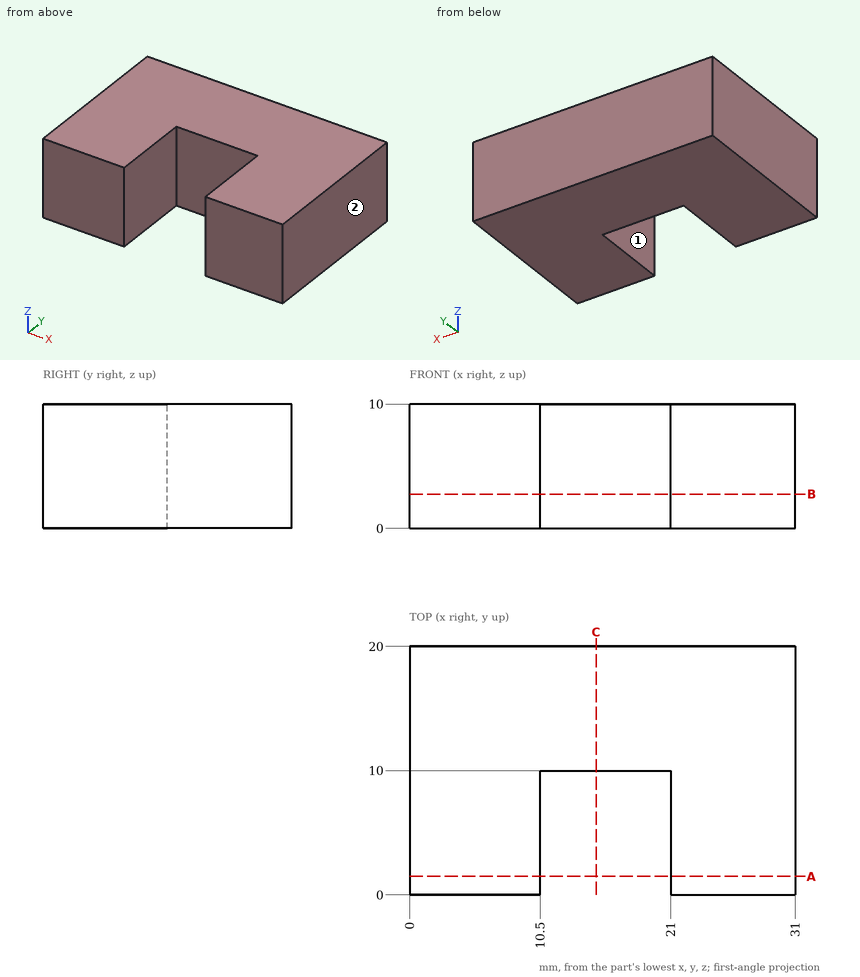
Verification items for this drawing (mm, ordinates from the low corner). A direction names the side the tool comes from. Give positions to 0.01 mm unless a question says otherwise; leave off trailing zeros. Order: outer loops, then holes, each group sorted by start corner. A loop starts at its lowest first (then second) coordinate and runs counter-clockwise, first axis right, second up.
1) Cross-section at A-A (y = 1.5). Record the boundary of the cut face in (x, z).
Results are:
outline: (0, 0) - (10.5, 0) - (10.5, 10) - (0, 10) - close; (21, 0) - (31, 0) - (31, 10) - (21, 10) - close
2) Cross-section at C-C (x = 15). Record the boundary of the cut face in (y, z), then the cut area to 3 significant figures.
Results are:
outline: (10, 0) - (20, 0) - (20, 10) - (10, 10) - close
area: 100 mm2
3) Material ranges on probe 1 along X at (y, z) = (6.5, 5); probe 2 along Y at (x, z) = (19.5, 4.5), recorded low to high.
Results are:
probe 1: x = 0 to 10.5, 21 to 31
probe 2: y = 10 to 20
4) Gauge pin test, flat end, axial feed: pin 1 (3 mm diameter, centred on x = 11.5, z = 3, fed in from -Y). Record the tip position at first contact, or that the pin passes through.
Results are:
pin 1: stops at y = 0
5) Cross-section at B-B (z = 2.75). Record the boundary of the cut face in (x, y).
Results are:
outline: (0, 0) - (10.5, 0) - (10.5, 10) - (21, 10) - (21, 0) - (31, 0) - (31, 20) - (0, 20) - close
6) Tool access check on the marked faces 1 and 2. Record the directions out of +Z, -Z, +X, -X, +Y, -Y that give a thin tool (end or side, any length) a straight path to the whole face; none if there is none.
Results are:
face 1: +Z, -Z, -Y
face 2: +Z, -Z, +X, +Y, -Y
